Geometry: see drawing. Coordinates: mm, zero at the bounding-box minimum. A direction names the side the tool comes from. Coordinates: 2 decimals unless noted, no trailing zeros. Order: outer loops, then holes, each group sorted by start corner. A loop starts at its lowest first (then second) coordinate and runs counter-clockwise, first axis right, second up. Notation, with made-up numbers: (3, -18) - (38, -18) arc R17 cw to (38, -14) - close; hole circle Ø7 at (34.25, 76). An arc over 180 degrees is marked (long way). Use a Markdown table: item, result. Add a question column.
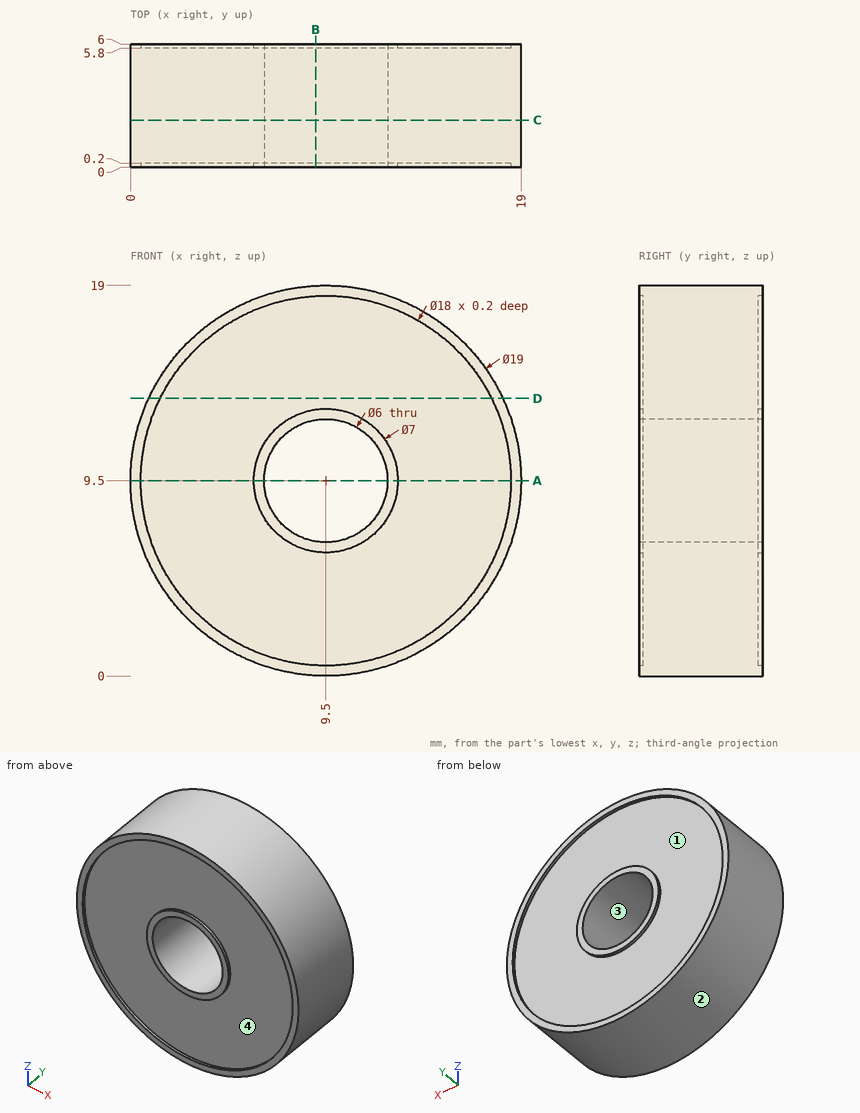
1) Contact query for flat-ended pins moving along their axis: P1, Ø9, axis at x = 12, z = 9.5, coming from the -Y side; P2, Ø1, axis at x = 4, y = 2.5, coming from the +Z side; P3, Ø1.5, axis at y = 4, z = 3, coming from the +X side. Output: stop coordinate, or through.
2) Cut plane A-A (z = 9.5). Return the cut outline in (x, y).
3) Cut plane D-D (z = 13.5). Return the cut outline in (x, y), and give its area (3 significant figures).
4) Reachability of the marked faces 3 and 4 from +Z, -Z, +X, -X, +Y, -Y: full face, straight path, thin tool, end or side. Return the list, or none.
5) Material intervals for L1, parallel to X at y = 0.1, z = 9.5; L2, parallel to Z at x = 9.5, y = 3.2, sorted ascending.
6) Cut plane C-C (y = 2.3). Return the cut outline in (x, z).
7) Cut plane B-B (x = 9). Return the cut outline in (y, z).
8) Pull-direction query (X, two-part tool) for the marked faces 1 and 2; classes: pulls with the +X half, pulls with the -X half, needs draft (parallel to the pull), parting line crosses it, or undercut.
Computed:
| question | item | result |
|---|---|---|
| 1 | P1 | stops at y = 0 |
| 1 | P2 | stops at z = 17.58 |
| 1 | P3 | stops at x = 17.06 |
| 2 | outline | (0, 0) - (0.5, 0) - (0.5, 0.2) - (6, 0.2) - (6, 0) - (6.5, 0) - (6.5, 6) - (6, 6) - (6, 5.8) - (0.5, 5.8) - (0.5, 6) - (0, 6) - close; (12.5, 0) - (13, 0) - (13, 0.2) - (18.5, 0.2) - (18.5, 0) - (19, 0) - (19, 6) - (18.5, 6) - (18.5, 5.8) - (13, 5.8) - (13, 6) - (12.5, 6) - close |
| 3 | outline | (0.88, 0) - (1.44, 0) - (1.44, 0.2) - (17.56, 0.2) - (17.56, 0) - (18.12, 0) - (18.12, 6) - (17.56, 6) - (17.56, 5.8) - (1.44, 5.8) - (1.44, 6) - (0.88, 6) - close |
| 3 | area | 97.0 mm2 |
| 4 | face 3 | +Y, -Y |
| 4 | face 4 | -Y |
| 5 | L1 | x = 0 to 0.5, 6 to 6.5, 12.5 to 13, 18.5 to 19 |
| 5 | L2 | z = 0 to 6.5, 12.5 to 19 |
| 6 | outline | circle Ø19 at (9.5, 9.5); hole circle Ø6 at (9.5, 9.5) |
| 7 | outline | (0, 0.01) - (6, 0.01) - (6, 0.51) - (5.8, 0.51) - (5.8, 6.04) - (6, 6.04) - (6, 6.54) - (0, 6.54) - (0, 6.04) - (0.2, 6.04) - (0.2, 0.51) - (0, 0.51) - close; (0, 12.46) - (6, 12.46) - (6, 12.96) - (5.8, 12.96) - (5.8, 18.49) - (6, 18.49) - (6, 18.99) - (0, 18.99) - (0, 18.49) - (0.2, 18.49) - (0.2, 12.96) - (0, 12.96) - close |
| 8 | face 1 | undercut |
| 8 | face 2 | parting line crosses it |
